Geometry: final body of the model. Coordinates: model frame, mm. A direction names the side the tool comes from. Round coordinates to 2 decimals unless told otherwise and drop trailing zeros. Loops run counter-clockwise (first coordinate to the right, second up) from the corner with the lowest first, then second, coordinate; pieces in that order, holes last. Notation, with made-up numbers: (67.5, 61.25) - (112.5, 61.25) arc R19 ccw to (112.5, 76.25) - close; hole circle Ø1 at (42, 7.25). An arc over 180 degrees is marked (long way). Write item = value, one per line. Start each with the question number.
Item 1: First-contact query: pin 1 (1.2 mm diameter, centred on x = -0.5, z = 41.5, fed in from +Y); pin 2 (0.8 mm diameter, centred on x = 0.5, z = 66, fed in from -Y); pin 3 (1.2 mm diameter, centred on x = 0, y = -27.5, fed in from +Z). Flat tips, straight axial feed; report the tip coordinate or a pass-through.
Item 2: Draft query along Z for faces 1 (the flat face through (0, 27.5, -15)), 2 (the cylindrical face through (-0.018, 5.745, 19.025)), 3 (the flat face through (0, -6.25, 46)). Return one class per face: pulls with the +Z half, pulls with the -Z half, needs draft (parallel to the pull), parting line crosses it, or undercut.
Item 3: Section A-A (z = 50.5). Return loops of the section in (x, y).
Item 4: Section D-D (x = -0.65). Count the separate pieces of the cut face and the enclosed holes in it, plus the area to 3 significant figures.
Item 5: Section C-C (z = 12.76). Return loops of the section in (x, y), plus the area to 3 significant figures.
Item 6: Access query for faces 4 (the flat face through (0, -9, -27)), 5 (the flat face through (0, -27, -7.507)), 6 (the flat face through (0, -30, -50)). Directions: +Z, -Z, +X, -X, +Y, -Y. A direction counts if a zero-diameter tool reaches every point of the face in a straight line with its end or side. Return the directions, or none.
Item 7: Section B-B (y = 0). Return loops of the section in (x, z).
Item 8: Line query: line 1 (Y direction, x = 0.65, z = 54.5); line 2 (Y direction, x = 0.6, z = 44); line 3 (Z direction, x = -0.6, y = 10.5). Output: solid intervals per line, ascending. Write a range as from..to.
from build123d import *

# Parameters (mm, degrees)
SKETCH1_R           = 1
SKETCH1_R_2         = 8.5
SKETCH1_W           = 10
SKETCH1_H           = 2.5
SKETCH1_W_2         = 38
SKETCH1_H_2         = 5
BOSS_EXTRUDE1_DEPTH = 1.25


with BuildPart() as part:
    # Sketch1 → Boss-Extrude1 (new, symmetric)
    with BuildSketch(Plane(origin=(0, 0, 0), x_dir=(0, 0, -1), z_dir=(1, 0, 0))):
        Polygon((-77.50700933, 25), (-77.50700933, -25), (-57.50700933, -25), (-57.50700933, -30), (-42.50700933, -30), (-42.50700933, -25), (-22.50700933, -25), (-22.50700933, -30), (-7.50700933, -30), (-7.50700933, -25), (7.50700933, -25), (7.50700933, -30), (22.50700933, -30), (22.50700933, -25), (42.50700933, -25), (42.50700933, -30), (57.50700933, -30), (57.50700933, -25), (77.50700933, -25), (77.50700933, 25), (57.50700933, 25), (57.50700933, 27.5), (42.50700933, 27.5), (42.50700933, 25), (22.50700933, 25), (22.50700933, 27.5), (7.50700933, 27.5), (7.50700933, 25), (-7.50700933, 25), (-7.50700933, 27.5), (-22.50700933, 27.5), (-22.50700933, 25), (-42.50700933, 25), (-42.50700933, 27.5), (-57.50700933, 27.5), (-57.50700933, 25), align=None)
        with Locations((-21.25, 8.75)):
            Circle(SKETCH1_R, mode=Mode.SUBTRACT)
        with Locations((-12.76, 0)):
            Circle(SKETCH1_R_2, mode=Mode.SUBTRACT)
        with Locations((-21.25, -8.75)):
            Circle(SKETCH1_R, mode=Mode.SUBTRACT)
        with Locations((12.76, 0)):
            Circle(SKETCH1_R_2, mode=Mode.SUBTRACT)
        with Locations((21.25, -8.75)):
            Circle(SKETCH1_R, mode=Mode.SUBTRACT)
        with Locations((21.25, 8.75)):
            Circle(SKETCH1_R, mode=Mode.SUBTRACT)
        with Locations((0, 17.5)):
            Rectangle(SKETCH1_W, SKETCH1_H, mode=Mode.SUBTRACT)
        with Locations((-46, -8.75)):
            Rectangle(SKETCH1_W_2, SKETCH1_H_2, mode=Mode.SUBTRACT)
        with Locations((0, -17.5)):
            Rectangle(SKETCH1_W, SKETCH1_H, mode=Mode.SUBTRACT)
        with Locations((-20, -17.5)):
            Rectangle(SKETCH1_W, SKETCH1_H, mode=Mode.SUBTRACT)
        with Locations((-20, 17.5)):
            Rectangle(SKETCH1_W, SKETCH1_H, mode=Mode.SUBTRACT)
        with Locations((-40, -17.5)):
            Rectangle(SKETCH1_W, SKETCH1_H, mode=Mode.SUBTRACT)
        with Locations((-40, 17.5)):
            Rectangle(SKETCH1_W, SKETCH1_H, mode=Mode.SUBTRACT)
        with Locations((-60, -17.5)):
            Rectangle(SKETCH1_W, SKETCH1_H, mode=Mode.SUBTRACT)
        with Locations((-60, 17.5)):
            Rectangle(SKETCH1_W, SKETCH1_H, mode=Mode.SUBTRACT)
        with Locations((20, -17.5)):
            Rectangle(SKETCH1_W, SKETCH1_H, mode=Mode.SUBTRACT)
        with Locations((20, 17.5)):
            Rectangle(SKETCH1_W, SKETCH1_H, mode=Mode.SUBTRACT)
        with Locations((40, -17.5)):
            Rectangle(SKETCH1_W, SKETCH1_H, mode=Mode.SUBTRACT)
        with Locations((40, 17.5)):
            Rectangle(SKETCH1_W, SKETCH1_H, mode=Mode.SUBTRACT)
        with Locations((60, -17.5)):
            Rectangle(SKETCH1_W, SKETCH1_H, mode=Mode.SUBTRACT)
        with Locations((60, 17.5)):
            Rectangle(SKETCH1_W, SKETCH1_H, mode=Mode.SUBTRACT)
        with Locations((46, 8.75)):
            Rectangle(SKETCH1_W_2, SKETCH1_H_2, mode=Mode.SUBTRACT)
        with Locations((-46, 0)):
            Rectangle(SKETCH1_W_2, SKETCH1_H_2, mode=Mode.SUBTRACT)
        with Locations((-46, 8.75)):
            Rectangle(SKETCH1_W_2, SKETCH1_H_2, mode=Mode.SUBTRACT)
        with Locations((46, -8.75)):
            Rectangle(SKETCH1_W_2, SKETCH1_H_2, mode=Mode.SUBTRACT)
        with Locations((0, 6.72)):
            Rectangle(SKETCH1_W, SKETCH1_H_2, mode=Mode.SUBTRACT)
        with Locations((46, 0)):
            Rectangle(SKETCH1_W_2, SKETCH1_H_2, mode=Mode.SUBTRACT)
    extrude(amount=BOSS_EXTRUDE1_DEPTH, both=True)


solid = part.part
Taken from the geometry:
q1.pin_1 = 25
q1.pin_2 = -25
q1.pin_3 = 57.51
q2.face_1 = needs draft
q2.face_2 = undercut
q2.face_3 = undercut
q3.outline = (-1.25, -30) - (1.25, -30) - (1.25, -11.25) - (-1.25, -11.25) - close; (-1.25, -6.25) - (1.25, -6.25) - (1.25, -2.5) - (-1.25, -2.5) - close; (-1.25, 2.5) - (1.25, 2.5) - (1.25, 6.25) - (-1.25, 6.25) - close; (-1.25, 11.25) - (1.25, 11.25) - (1.25, 27.5) - (-1.25, 27.5) - close
q4.separate_pieces = 1
q4.enclosed_holes = 27
q4.area = 6,190 mm^2
q5.outline = (-1.25, -30) - (1.25, -30) - (1.25, -8.5) - (-1.25, -8.5) - close; (-1.25, 8.5) - (1.25, 8.5) - (1.25, 27.5) - (-1.25, 27.5) - close
q5.area = 101 mm^2
q6.face_4 = +X, -X
q6.face_5 = +X, -X, -Y
q6.face_6 = +Z, -Z, +X, -X, -Y
q7.outline = (-1.25, -77.51) - (1.25, -77.51) - (1.25, -65) - (-1.25, -65) - close; (-1.25, -27) - (1.25, -27) - (1.25, -21.26) - (-1.25, -21.26) - close; (-1.25, -4.26) - (1.25, -4.26) - (1.25, 4.26) - (-1.25, 4.26) - close; (-1.25, 21.26) - (1.25, 21.26) - (1.25, 27) - (-1.25, 27) - close; (-1.25, 65) - (1.25, 65) - (1.25, 77.51) - (-1.25, 77.51) - close
q8.line_1 = -30..-11.25, -6.25..-2.5, 2.5..6.25, 11.25..27.5
q8.line_2 = -30..-18.75, -16.25..-11.25, -6.25..-2.5, 2.5..6.25, 11.25..16.25, 18.75..27.5
q8.line_3 = -77.51..-65, -27..27, 65..77.51
